Here's how the part is built. I have some questions about the finished solid (model axes, mm). A direction names the side the tool comes from. Coordinates: 2 decimals unless noted, no trailing zeros. Loops run counter-clockwise (first coordinate to the right, second up) from the corner with the lowest first, then second, coordinate; pieces in that order, holes last. Notation, with made-up numbers: (13.5, -31.75) -> (34.5, -31.75) arc R26 ccw to (34.5, -15.75) -> close; hole circle Ø1 at (81, 14). An arc over 180 degrees is marked (long way). Answer as a JSON object with one key per item and string values. Group by question number.
Q1. On a 3-axis mill with a long thin cutter (end or side, diameter ignored), from which of +Z, -Z, +X, -X, +Y, -Y can I reach the whole of each face in a straight line? I mean faces 1 (the flat face through (10, 7, 4)), 2 (the cylindrical face through (1.004, 6.071, 4.522)), 3 (the conical face through (0.89, 2.97, 4)). Say none if no direction works.
Q2. I need wall thicknesses on line 1 (X direction, y = 4, z = 0); line 2 (X direction, y = 5.25, z = 0); line 3 (Z direction, x = -0.25, y = 6). Which ranges of each line are inside material? Lowest first, please.
Q3. I'm going to push flat-ended pins straight in: pin 1 (3.5 mm diameter, centred on x = -2.5, z = -2.5, fed in from +Y); pin 2 (6 mm diameter, centred on x = 3, z = -1, fed in from -Y); pin 3 (1 mm diameter, centred on y = 3.5, z = 8, fed in from -X); pin 4 (1 mm diameter, centred on x = -7, y = 3, fed in from +Z). Where does each tip first touch, or does it pass through?
Q4. I want a section at A-A on y = 3. Write out the boundary of the cut face in (x, z).
Q5. Thinking about a two-plate mould opening in Y: for faces 4 (the flat face through (4.3, 0.5, 4.3)), 5 (the flat face through (-5, 0, 5)), 6 (the conical face through (0.99, 3.36, 4.46)), which applies, released by +Y, released by -Y, zero draft, split by the parting line, or undercut?
```python
from build123d import *


with BuildPart() as part:
    # 草图1 → 旋转1 (revolve)
    with BuildSketch(Plane.XY):
        with BuildLine():
            Line((-10.5, 0), (-5.769439135, 0))
            ThreePointArc((-5.769439135, 0), (-5.259121106, 0.133562425), (-4.879665027, 0.5))
            Line((-4.879665027, 0.5), (-4.315491633, 0))
            Line((-4.315491633, 0), (-3.565536978, 0.06561253))
            Line((-3.565536978, 0.06561253), (-4.315491633, 0.5))
            Line((-4.315491633, 0.5), (-3.965536978, 4.5))
            Line((-3.965536978, 4.5), (-3.565536978, 4.5))
            Line((-3.565536978, 4.5), (-3, 5.928571429))
            Line((-3, 5.928571429), (-3.680070479, 6.404761905))
            Line((-3.680070479, 6.404761905), (-4.632451432, 6.404761905))
            Line((-4.632451432, 6.404761905), (-4.632451432, 5.747213595))
            ThreePointArc((-4.632451432, 5.747213595), (-4.867701612, 5.244464966), (-4.432451432, 4.9))
            Line((-4.432451432, 4.9), (-4.77365722, 1))
            Line((-4.77365722, 1), (-5.480764001, 1))
            Line((-5.480764001, 1), (-5.769439135, 0.5))
            Line((-5.769439135, 0.5), (-10.1, 0.5))
            Line((-10.1, 0.5), (-10.5, 0.9))
            Line((-10.5, 0.9), (-10.5, 7))
            Line((-10.5, 7), (-11, 7))
            Line((-11, 7), (-11, 0.5))
            Line((-11, 0.5), (-10.5, 0))
        make_face()
    revolve(axis=Axis((0, 5.977335763, 0), (0, -1, 0)))


solid = part.part
```
Result set:
{
 "1": {"face 1": "+Z, -Z, +X, -X, +Y", "face 2": "+Y", "face 3": "none"},
 "2": {"line 1": "x = -11 to -10.5, -4.51 to -4.01, 4.01 to 4.51, 10.5 to 11", "line 2": "x = -11 to -10.5, -4.87 to -3.27, 3.27 to 4.87, 10.5 to 11", "line 3": "z = -11 to -10.5, -4.63 to -3.09, 3.09 to 4.63, 10.5 to 11"},
 "3": {"pin 1": "stops at y = 6.4", "pin 2": "stops at y = 0", "pin 3": "stops at x = -8.05", "pin 4": "stops at z = 8.87"},
 "4": {"outline": "circle Ø22 at (0, 0); circle Ø9.2 at (0, 0); hole circle Ø21 at (0, 0); hole circle Ø8.19 at (0, 0)"},
 "5": {"face 4": "released by +Y", "face 5": "released by -Y", "face 6": "undercut"}
}
